Geometry: see drawing. Coordinates: mm, zero at the bounding-box minimum. A direction names the side the tool comes from. Coordinates: 2 decimals unless noted, no trailing zeros. Loops run counter-clockwise (first coordinate to the right, second up) from the corner with the lowest first, then second, coordinate; pieces in that order, holes last. Notation, with made-up numbers: (26.25, 76) - (73.25, 76) arc R27 ccw to (73.25, 108) - close; hole circle Ø6 at (42.25, -20.75). An arc over 180 degrees is marked (long way). Use a Markdown table: item, result. Add a question column.
1. Section query B-B on x = 23.5. Return the cut outline in (y, z).
2. Section query C-C on z = 20. Return the cut outline in (x, y) (1 decimal), then the cut area to 3 significant figures.
3. Draft query along Z for the marked faces 3, 4 and 5. Return one class per face: released by +Z, released by -Z, zero draft, split by the parting line, or undercut.
4. Access query for the marked faces 1 and 2. Directions: +Z, -Z, +X, -X, +Y, -Y. A direction counts if a zero-diameter tool reaches every point of the face in a straight line with its end or side. Return the directions, or none.
5. Ray query, L1, parallel to X at y = 14, z = 22 (1 decimal); L2, parallel to Z at x = 22, y = 9.25 (1 decimal); L3, parallel to X at y = 2, z = 32 (1 decimal). Return the intervals inside material, ascending. Write a range as [from, to].
6. Section query D-D on x = 14. Return the cut outline in (y, z) (1 decimal).
7. Contact query for flat-ended pins moving along their axis: P1, Ø10, axis at x = 10.5, z = 25.5, coming from the -Y side; P2, Ø4, axis at y = 9, z = 8, coming from the +X side; P3, Ø5, axis at x = 21.4, z = 21.4, coming from the -Y side; P4, Ø12, axis at x = 20.5, z = 28, coming from the -Y side. Output: stop coordinate, or through.
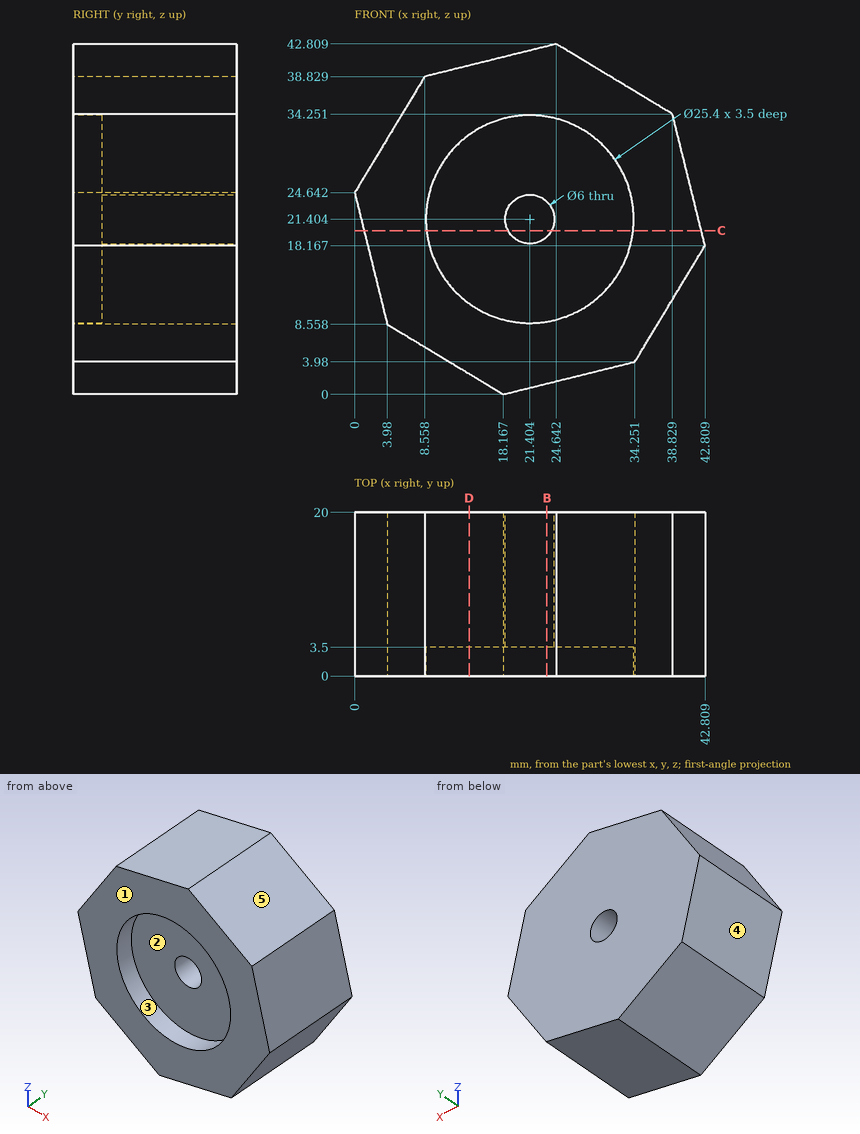
Resolved:
| question | item | result |
|---|---|---|
| 1 | outline | (0, 1.32) - (20, 1.32) - (20, 19.26) - (3.5, 19.26) - (3.5, 8.88) - (0, 8.88) - close; (0, 33.93) - (3.5, 33.93) - (3.5, 23.55) - (20, 23.55) - (20, 42.53) - (0, 42.53) - close |
| 2 | outline | (1.1, 0) - (8.8, 0) - (8.8, 3.5) - (18.8, 3.5) - (18.8, 20) - (1.1, 20) - close; (24.1, 3.5) - (34, 3.5) - (34, 0) - (42.4, 0) - (42.4, 20) - (24.1, 20) - close |
| 2 | area | 648 mm² |
| 3 | face 3 | undercut |
| 3 | face 4 | released by -Z |
| 3 | face 5 | released by +Z |
| 4 | face 1 | +Z, -Z, +X, -X, -Y |
| 4 | face 2 | -Y |
| 5 | L1 | [0.7, 18.5], [24.3, 41.9] |
| 5 | L2 | [0.9, 18.5], [24.3, 42.2] |
| 5 | L3 | [4.4, 14.4], [28.4, 39.4] |
| 6 | outline | (0, 2.5) - (20, 2.5) - (20, 40.2) - (0, 40.2) - (0, 31.7) - (3.5, 31.7) - (3.5, 11.1) - (0, 11.1) - close |
| 7 | P1 | y = 0 |
| 7 | P2 | x = 37.88 |
| 7 | P3 | through |
| 7 | P4 | y = 3.5 |
